Can you work these out from the model? Positions are in its coordinate system, mm. A direction names the side the tool comes from. Round coordinates to 2 decimals unless told otherwise and drop trailing zeros. Order: outer loops, then holes, each group sorted by start corner. A loop starts at its lowest first (then second) coordinate and runs counter-clockwise, first axis right, second up.
Q1. If we section it at D-D (x = 4.75): Please give me the cut outline in (y, z), plus the area to 3 significant figures.
Q2. We'd pull the mould along X, two halves only. Please class faces 1 (the face through (6.6, 11, 3)), 2 (the face through (15, 9.5, 3)), 3 (the face through (18.35, -3, 3)), 4 (the face through (15.835, 2.05, 3.154)): pulls with the +X half, pulls with the -X half, needs draft (parallel to the pull), parting line crosses it, or undercut.
Q3. If we section it at B-B (x = 15): Please give me the cut outline in (y, z), plus the area to 3 significant figures.
Q4. For faces 5 (the face through (18, 16, 0.7)), 6 (the face through (14.56, 14.26, 3.24)), 7 (the face through (1.65, -2, 2)), 8 (the face through (11.05, -2, 2)), which set-ups out of +Z, -Z, +X, -X, +Y, -Y let a thin tool reach every point of the face, with its end or its side?
Q5. Will these pins go through, and if not, where does the flat tip stop? P1, Ø1, axis at y = -1.5, z = 3.5, coming from the +X side; P2, Ø5, axis at x = 12, y = 4, coming from the +Z side; P3, Ø10.5, axis at x = 9.5, y = 16.5, coming from the +Z side; P4, Ø3, axis at x = 12.5, y = 7.5, coming from the -Z side.
Q6. If I drill on line 1 (X direction, y = -2, z = 4.25); line 2 (Y direction, x = 18.1, z = 3.2); line 3 (Y direction, x = 5.25, z = 2) (3 decimals), over which ranges is the centre line in solid material (lowest first)?
Q7. If we section it at A-A (z = 3.2): Count the separate pieces of the cut face and the enclosed holes in it, plus the area to 3 significant figures.
from build123d import *

# Parameters (mm, degrees)
SKETCH_1_W               = 20
SKETCH_1_H               = 10.2
SKETCH_1_R               = 1.175
EXTRUDE_1_DEPTH          = 6.4
CUT_EXTRUDE_1_DEPTH      = 1
CUT_EXTRUDE_1_DEPTH_BACK = 7.4
FILLET_1_R               = 0.1
FILLET_2_R               = 0.5
SKETCH_8_R               = 1.175
EXTRUDE_5_DEPTH          = 0.1
CHAMFER_1_SIZE           = 0.2
SKETCH_3_W               = 0.6
SKETCH_3_H               = 3.9
EXTRUDE_2_DEPTH          = 1.6
SKETCH_9_R               = 0.8
CUT_EXTRUDE_2_DEPTH      = 19.35
CHAMFER_2_SIZE           = 0.2
SKETCH_5_R               = 1
EXTRUDE_3_DEPTH          = 2.5
EXTRUDE_6_DEPTH          = 2.5
FILLET_3_R               = 0.3


with BuildPart() as part:
    # Sketch 1 → Extrude 1 (new body)
    with BuildSketch(Plane.XY):
        with Locations((10, 5.1)):
            Rectangle(SKETCH_1_W, SKETCH_1_H)
        with Locations((5.25, 2.5)):
            Circle(SKETCH_1_R, mode=Mode.SUBTRACT)
        with Locations((14.75, 2.5)):
            Circle(SKETCH_1_R, mode=Mode.SUBTRACT)
    extrude(amount=EXTRUDE_1_DEPTH)

    # Sketch 7 → Cut-Extrude 1 (cut, two sides)
    with BuildSketch(Plane.XY.offset(6.4)) as cut_extrude_1_sk:
        Polygon((20, 9.5), (10, 9.5), (9.412630258, 10.2), (20, 10.2), align=None)
    extrude(amount=CUT_EXTRUDE_1_DEPTH, mode=Mode.SUBTRACT)
    extrude(cut_extrude_1_sk.sketch, amount=-CUT_EXTRUDE_1_DEPTH_BACK, mode=Mode.SUBTRACT)

    # Fillet 1
    fillet_1_edges = [part.edges().sort_by_distance(p)[0] for p in [
        (9.412630258, 10.2, 3.2),
        (10, 9.5, 3.2),
    ]]
    fillet(fillet_1_edges, radius=FILLET_1_R)

    # Fillet 2
    fillet_2_edges = [part.edges().sort_by_distance(p)[0] for p in [
        (20, 9.5, 3.2),
        (0, 10.2, 3.2),
        (20, 0, 3.2),
        (0, 0, 3.2),
    ]]
    fillet(fillet_2_edges, radius=FILLET_2_R)

    # Sketch 8 → Extrude 5 (add)
    with BuildSketch(Plane.XY.offset(6.4)):
        with BuildLine():
            Line((4, 2.5), (4, 0))
            Line((4, 0), (6.5, 0))
            Line((6.5, 0), (6.5, 2.5))
            ThreePointArc((6.5, 2.5), (5.25, 3.75), (4, 2.5))
        make_face()
        with Locations((5.25, 2.5)):
            Circle(SKETCH_8_R, mode=Mode.SUBTRACT)
        with BuildLine():
            Line((13.5, 2.5), (13.5, 0))
            Line((13.5, 0), (16, 0))
            Line((16, 0), (16, 2.5))
            ThreePointArc((16, 2.5), (14.75, 3.75), (13.5, 2.5))
        make_face()
        with Locations((14.75, 2.5)):
            Circle(SKETCH_8_R, mode=Mode.SUBTRACT)
    extrude_5 = extrude(amount=EXTRUDE_5_DEPTH)

    # Mirror 1: Extrude 5 across plane
    add(extrude_5.mirror(Plane.XY.offset(3.2)))

    # Chamfer 1
    chamfer_1_edges = [part.edges().sort_by_distance(p)[0] for p in [
        (6.5, 0, -0.05),
        (4, 0, -0.05),
        (16, 0, -0.05),
        (13.5, 0, -0.05),
        (4, 0, 6.45),
        (6.5, 0, 6.45),
        (13.5, 0, 6.45),
        (16, 0, 6.45),
    ]]
    chamfer(chamfer_1_edges, length=CHAMFER_1_SIZE)

    # Sketch 3 → Extrude 2 (add, symmetric)
    with BuildSketch(Plane.XY.offset(3.2)):
        with Locations((1.95, -1.95)):
            Rectangle(SKETCH_3_W, SKETCH_3_H)
        with Locations((10.75, -1.95)):
            Rectangle(SKETCH_3_W, SKETCH_3_H)
        with Locations((18.05, -1.95)):
            Rectangle(SKETCH_3_W, SKETCH_3_H)
    extrude(amount=EXTRUDE_2_DEPTH, both=True)

    # Sketch 9 → Cut-Extrude 2 (cut, through all)
    with BuildSketch(Plane.ZY.offset(-1.65)):
        with Locations((3.2, -1.95)):
            Circle(SKETCH_9_R)
    extrude(amount=-CUT_EXTRUDE_2_DEPTH, mode=Mode.SUBTRACT)

    # Chamfer 2
    chamfer_2_edges = [part.edges().sort_by_distance(p)[0] for p in [
        (1.95, -3.9, 1.6),
        (1.95, -3.9, 4.8),
        (10.75, -3.9, 1.6),
        (10.75, -3.9, 4.8),
        (18.05, -3.9, 1.6),
        (18.05, -3.9, 4.8),
    ]]
    chamfer(chamfer_2_edges, length=CHAMFER_2_SIZE)



with BuildPart() as body_2:
    # Sketch 5 → Extrude 3 (new body, symmetric)
    with BuildSketch(Plane.XY.offset(3.2)):
        with BuildLine():
            Line((21.3, 18), (21.3, 16.267087306))
            Line((21.3, 16.267087306), (21.3, 16.163171396))
            Line((21.3, 16.163171396), (3.1, 11.020209549))
            Line((3.1, 11.020209549), (3.1, 10.193829773))
            Line((3.1, 10.193829773), (2.9, 10.2))
            Line((2.9, 10.2), (2.9, 11.171525305))
            Line((2.9, 11.171525305), (17.5, 15.297197995))
            Line((17.5, 15.297197995), (17.5, 18))
            ThreePointArc((17.5, 18), (19.4, 19.9), (21.3, 18))
        make_face()
        with Locations((19.4, 18)):
            Circle(SKETCH_5_R, mode=Mode.SUBTRACT)
    extrude(amount=EXTRUDE_3_DEPTH, both=True)


with BuildPart() as part_1:
    add(part.part)

    add(body_2.part)  # Extrude 6 merges body 2
    # Sketch 10 → Extrude 6 (add, symmetric)
    with BuildSketch(Plane.XY.offset(3.2)):
        with BuildLine():
            Line((6.6, 11.4), (6.6, 10.2))
            Line((6.6, 10.2), (8.6, 10.2))
            Line((8.6, 10.2), (8.6, 11.4))
            ThreePointArc((8.6, 11.4), (7.6, 12.4), (6.6, 11.4))
        make_face()
    extrude(amount=EXTRUDE_6_DEPTH, both=True)

    # Fillet 3
    fillet_3_edges = [part_1.edges().sort_by_distance(p)[0] for p in [
        (21.3, 16.163171396, 3.2),
    ]]
    fillet(fillet_3_edges, radius=FILLET_3_R)


solid = part_1.part
Solution:
1. outline: (0, -0.1) - (1.44, -0.1) - (1.44, 6.5) - (0, 6.5) - close; (3.56, -0.1) - (3.65, -0.1) - (3.65, 0) - (10.2, 0) - (10.2, 6.4) - (3.65, 6.4) - (3.65, 6.5) - (3.56, 6.5) - close; (11.49, 0.7) - (11.69, 0.7) - (11.69, 5.7) - (11.49, 5.7) - close
1. area: 53.0 mm2
2. face 1: undercut
2. face 2: needs draft
2. face 3: pulls with the +X half
2. face 4: undercut
3. outline: (0, -0.1) - (1.35, -0.1) - (1.35, 6.5) - (0, 6.5) - close; (3.65, -0.1) - (3.72, -0.1) - (3.72, 0) - (9.5, 0) - (9.5, 6.4) - (3.72, 6.4) - (3.72, 6.5) - (3.65, 6.5) - close; (14.38, 0.7) - (14.59, 0.7) - (14.59, 5.7) - (14.38, 5.7) - close
3. area: 47.4 mm2
4. face 5: -Z, +X, -X, +Y
4. face 6: +Z, -Z, +X
4. face 7: +Z, -Z, -X, -Y
4. face 8: +Z, -Z, -Y
5. P1: stops at x = 18.35
5. P2: stops at z = 6.5
5. P3: stops at z = 5.7
5. P4: stops at z = 0
6. line 1: x = 1.65 to 2.25, 10.45 to 11.05, 17.75 to 18.35
6. line 2: y = -3.9 to -2.75, -1.15 to 9.5, 15.26 to 19.39
6. line 3: y = 0 to 1.325, 3.675 to 10.2, 11.628 to 11.836
7. separate pieces: 4
7. enclosed holes: 4
7. area: 211 mm2
